Job drawing, mm, ordinate dimensions from the low corner. One solid piece. A direction names the side the tool comes from. Coordinates: 2 decimals unless noted, no trailing zeros. Order: outer loops, then holes, each group sorted by start corner. A loop starts at its lowest first (then second) coordinate and runs counter-clockwise, first axis right, second up. Notation, with made-up numbers: (27, 63.5) - (54, 63.5) arc R27 ccw to (54, 83.5) - close; hole circle Ø9 at (19, 30.5). An arc over 180 degrees is marked (long way). Write each question's results on one line, items separated by ' | '. Start each with the question number.
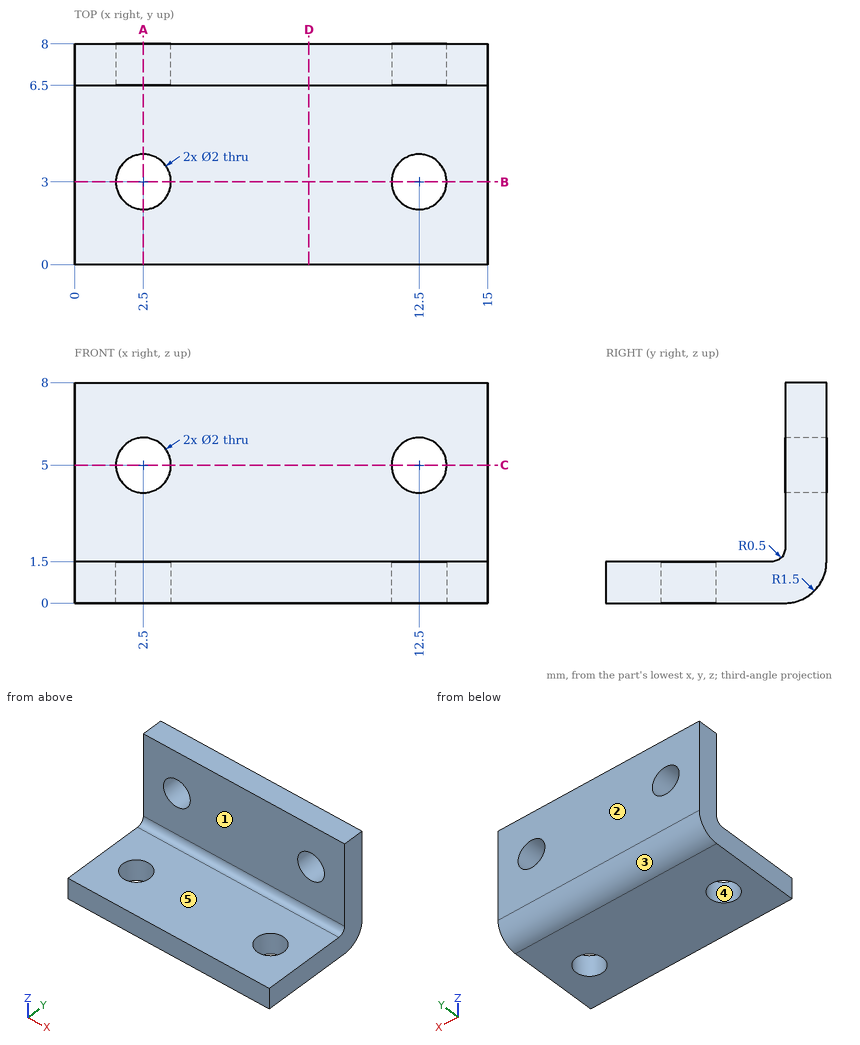
Item 1: Slice it at B-B (y = 3). Write the cut outline in (x, z), then the cut area to 3 significant figures.
Item 2: Flat gauge pins, fed straight in: P1, Ø1.2, axis at x = 12.5, z = 5, coming from the +Y side; P2, Ø3, axis at x = 5.5, z = 4.5, coming from the -Y side; P3, Ø3, axis at x = 5, y = 4.5, coming from the +Z side. Where does each tip first touch, or does it go through?
Item 3: Slice it at D-D (x = 8.5). Write the cut outline in (y, z), then the cut area to 3 significant figures.
Item 4: Slice it at A-A (x = 2.5). Write the cut outline in (y, z), then the cut area to 3 significant figures.
Item 5: Which spindle directions (+Z, -Z, +X, -X, +Y, -Y) get a long thin tool onto all of the face, cutting with end or side? Do the marked faces 1 and 2. Say none if no direction does.
Item 6: Probe probe 1 along X at (y, z) = (7.5, 5.5); probe 2 along Y at (x, z) = (2, 3); probe 3 along Z at (x, y) = (14.25, 2). List the from-to ranges inside material, lowest first.
Item 7: Slice it at C-C (z = 5). Write the cut outline in (x, y).
Item 8: Pull direction Y, two halves, no side cores. Call the marked faces 3, 4 and 5: released by +Y, released by -Y, zero draft, split by the parting line, or undercut.
Resolved:
1) outline: (0, 0) - (1.5, 0) - (1.5, 1.5) - (0, 1.5) - close; (3.5, 0) - (11.5, 0) - (11.5, 1.5) - (3.5, 1.5) - close; (13.5, 0) - (15, 0) - (15, 1.5) - (13.5, 1.5) - close | area: 16.5 mm^2
2) P1: through | P2: y = 6.5 | P3: z = 1.5
3) outline: (0, 0) - (6.5, 0) arc R1.5 ccw to (8, 1.5) - (8, 8) - (6.5, 8) - (6.5, 2) arc R0.5 cw to (6, 1.5) - (0, 1.5) - close | area: 21.3 mm^2
4) outline: (0, 0) - (2, 0) - (2, 1.5) - (0, 1.5) - close; (4, 0) - (6.5, 0) arc R1.5 ccw to (8, 1.5) - (8, 4) - (6.5, 4) - (6.5, 2) arc R0.5 cw to (6, 1.5) - (4, 1.5) - close; (6.5, 6) - (8, 6) - (8, 8) - (6.5, 8) - close | area: 15.3 mm^2
5) face 1: +Z, +X, -X, -Y | face 2: +Z, -Z, +X, -X, +Y
6) probe 1: 0 to 1.63, 3.37 to 11.63, 13.37 to 15 | probe 2: 6.5 to 8 | probe 3: 0 to 1.5
7) outline: (0, 6.5) - (1.5, 6.5) - (1.5, 8) - (0, 8) - close; (3.5, 6.5) - (11.5, 6.5) - (11.5, 8) - (3.5, 8) - close; (13.5, 6.5) - (15, 6.5) - (15, 8) - (13.5, 8) - close
8) face 3: released by +Y | face 4: undercut | face 5: zero draft
